from build123d import *

# Parameters (mm, degrees)
F1_DEPTH = 76.2
F2_R     = 10.043167
F2_R_2   = 9.191604
F3_DEPTH = 25.4


with BuildPart() as f1:
    # F0 (on Front) → F1 (new body)
    with BuildSketch(Plane.XZ):
        with BuildLine():
            Line((-63.273966, 17.029652), (-63.273966, 10.570128))
            Line((-63.273966, 10.570128), (-12.772239, 10.570128))
            ThreePointArc((-12.772239, 10.570128), (7.340368, 25.418198), (27.452976, 10.570128))
            Line((27.452976, 10.570128), (77.954703, 10.570128))
            Line((77.954703, 10.570128), (77.954703, 17.029652))
            Line((77.954703, 17.029652), (35.380573, 17.029652))
            ThreePointArc((35.380573, 17.029652), (7.340368, 34.793164), (-20.699836, 17.029652))
            Line((-20.699836, 17.029652), (-63.273966, 17.029652))
        make_face()
    extrude(amount=F1_DEPTH)

    # F2 (on face) → F3 (cut)
    with BuildSketch(Plane.XY.offset(17.029652)):
        with Locations((-45.073345, -41.106056)):
            Circle(F2_R)
        with Locations((57.104558, -41.106056)):
            Circle(F2_R_2)
    extrude(amount=-F3_DEPTH, mode=Mode.SUBTRACT)


solid = f1.part
The listing builds one solid part. Answer for the finished solid, in the listing's coordinates (mm). A direction names the side the tool comes from. Round coordinates to 2 decimals unless told otherwise and drop trailing zeros. Write each loop counter-clockwise with the first axis right and the second up, starting at its lowest first coordinate (ties: lowest second). Pieces come first, ordered by that corner, then holes. Notation, with made-up numbers: (37.25, 16) - (64.25, 16) arc R23 ccw to (64.25, 47) - close; hole circle Ø11 at (69.5, -36). An arc over 180 degrees is marked (long way). Use one line per item in the form item = value. Start each with the question number.
Item 1: Flat-ended cylindrical pins translate along their axes: pin 1 Ø13 at (x, y) = (-32, -30) entering from +Z; pin 2 Ø3 at (y, z) = (-67, 25.5) entering from +X. Find the tip coordinate at first contact, or state that the pin passes through.
Item 2: A cutting plane is placed at D-D (z = 19.5). Write down the section's boundary in (x, y), plus the area to 3 significant figures.
Item 3: A cutting plane is placed at C-C (y = -46.5). Write down the section's boundary in (x, z).
Item 4: Determine the mould class of faces 1 (the flat face through (-33, -38, 10.57)), 2 (the flat face through (-63.274, -38, 14)), 3 (the cylindrical face through (49.81, -46.7, 13.85)), 4 (the flat face through (77.955, -38, 14)) for opening direction X: +X half, -X half, draft (parallel to the pull), parting line (faces both ways), or undercut.
Item 5: A tool of negligible diameter and unlimited length cuts with its end or side. For faces 5 (the cylindrical face through (7.83, -37.57, 34.79)), 6 (the flat face through (-42, -29, 17.03)), 7 (the flat face through (57, -29, 17.03)), from which of +Z, -Z, +X, -X, +Y, -Y can it reach the whole face along a straight path? Write none if from no direction.
Item 6: A cutting plane is placed at B-B (x = 52). Write down the section's boundary in (y, z), plus the area to 3 significant figures.
Item 7: Find the intervals of material crossed by line 1 (Z direction, x = 49.5, y = -29); line 2 (X direction, y = -34.5, z = 16.75); line 3 (X direction, y = -72.5, z = 19), in increasing order. Write a range as [from, to].
Item 8: A cutting plane is placed at A-A (z = 13.75). Write down the section's boundary in (x, y), plus the area to 3 significant figures.
The answers:
q1.pin_1 = 17.03
q1.pin_2 = 30.86
q2.outline = (-19.39, -76.2) - (-7.29, -76.2) - (-7.29, 0) - (-19.39, 0) - close; (21.97, -76.2) - (34.07, -76.2) - (34.07, 0) - (21.97, 0) - close
q2.area = 1,840 mm^2
q3.outline = (-63.27, 10.57) - (-53.55, 10.57) - (-53.55, 17.03) - (-63.27, 17.03) - close; (-36.6, 10.57) - (-12.77, 10.57) arc R21.05 cw to (27.45, 10.57) - (49.66, 10.57) - (49.66, 17.03) - (35.38, 17.03) arc R31.01 ccw to (-20.7, 17.03) - (-36.6, 17.03) - close; (64.55, 10.57) - (77.95, 10.57) - (77.95, 17.03) - (64.55, 17.03) - close
q4.face_1 = draft
q4.face_2 = -X half
q4.face_3 = undercut
q4.face_4 = +X half
q5.face_5 = +Z, +Y, -Y
q5.face_6 = +Z, -X, +Y, -Y
q5.face_7 = +Z, +X, +Y, -Y
q6.outline = (-76.2, 10.57) - (-48.75, 10.57) - (-48.75, 17.03) - (-76.2, 17.03) - close; (-33.46, 10.57) - (0, 10.57) - (0, 17.03) - (-33.46, 17.03) - close
q6.area = 393 mm^2
q7.line_1 = [10.57, 17.03]
q7.line_2 = [-63.27, -52.64], [-37.51, -9.68], [24.36, 50.71], [63.5, 77.95]
q7.line_3 = [-19.68, -7.79], [22.47, 34.36]
q8.outline = (-63.27, -76.2) - (-11.5, -76.2) - (-11.5, 0) - (-63.27, 0) - close; (26.18, -76.2) - (77.95, -76.2) - (77.95, 0) - (26.18, 0) - close; hole circle Ø20.09 at (-45.07, -41.11); hole circle Ø18.38 at (57.1, -41.11)
q8.area = 7,310 mm^2
